Can you work these out from the model? Positions are in its coordinate system, mm. A direction names the side the tool comes from. Coordinates: 2 decimals unless noted, no trailing zeros. Order: outer loops, then holes, each group sorted by start corner. A loop starts at its lowest first (then second) coordinate and runs counter-clockwise, first axis right, second up. Notation, with made-up numbers: (66, -2) -> (108, -2) arc R16 ccw to (108, 5) -> close; hole circle Ø3 at (-32.75, 18). An arc over 180 degrees is marked (long way). Write item = value, one per line.
```python
from build123d import *

# Parameters (mm, degrees)
BOSS_EXTRUDE1_DEPTH = 17
CUT_EXTRUDE1_DEPTH  = 31
SKETCH3_W           = 12.47
SKETCH3_H           = 10.75
CUT_EXTRUDE2_REACH  = 37.239
SKETCH6_W           = 10
SKETCH6_H           = 10.75
SKETCH7_R           = 4
CUT_EXTRUDE3_DEPTH  = 31


with BuildPart() as part:
    # Sketch1 → Boss-Extrude1 (new body)
    with BuildSketch(Plane.XY):
        Polygon((0, 0), (0, 11.1), (5.04, 11.1), (5.04, -5.9), (1.928970145, -13.9), (-4.358645915, -16.03435805), (-26.37555014, -13.036971131), (-26.37555014, 11.1), (-21.33555014, 11.1), (-21.33555014, 0), align=None)
    extrude(amount=BOSS_EXTRUDE1_DEPTH)

    # Sketch2 → Cut-Extrude1 (cut, symmetric)
    with BuildSketch(Plane.ZY):
        Polygon((8.228054067, 11.1), (17, 11.1), (17, 12.88110255), (0, 12.88110255), (0, 11.1), align=None)
        with BuildLine():
            ThreePointArc((0, 0), (2.28131811, 6.908525055), (8.228054067, 11.1))
            Line((8.228054067, 11.1), (0, 11.1))
            Line((0, 11.1), (0, 0))
        make_face()
        Polygon((13.228054067, 10.512247596), (17, 6.76), (17, 11.1), (8.228054067, 11.1), align=None)
    extrude(amount=CUT_EXTRUDE1_DEPTH, both=True, mode=Mode.SUBTRACT)

    # Cut-Sweep1: sweep along a path in Sketch5
    with BuildLine(Plane.XY.offset(7)) as cut_sweep1_path:
        Line((-9.535960256, -15.329517164), (-6.500512954, -6.687083497))
    # Sketch3 → Cut-Sweep1 (sweep, cut)
    with BuildSketch(Plane(origin=(-2.222513014, -16.325171724, 0), x_dir=(-0.990859776111597, 0.13489590091650622, 0), z_dir=(-0.13489590091650622, -0.990859776111597, 0))):
        with Locations((12.41083774, -9.115)):
            Rectangle(SKETCH3_W, SKETCH3_H)
    sweep(path=cut_sweep1_path.line, mode=Mode.SUBTRACT)

    # Cut-Extrude2: up to this plane
    cut_extrude2_end = Plane(origin=(-8.680240671, -16.455383538, 3.74), z_dir=(-0.943497125175066, 0.33138070973788714, 0))
    # Sketch6 → Cut-Extrude2 (cut, up to the surface)
    with BuildSketch(Plane(origin=(0, 0, 0), x_dir=(1, 0, 0), z_dir=(0, 1, 0)), mode=Mode.PRIVATE) as cut_extrude2_sk1:
        with Locations((-8.42, -9.115)):
            Rectangle(SKETCH6_W, SKETCH6_H)
    cut_extrude2_tool1 = split(extrude(cut_extrude2_sk1.sketch, amount=-CUT_EXTRUDE2_REACH, mode=Mode.PRIVATE), bisect_by=cut_extrude2_end, keep=Keep.BOTH, mode=Mode.PRIVATE)
    add(cut_extrude2_tool1.solids().sort_by_distance((-8.42, 0, 9.115))[0], mode=Mode.SUBTRACT)

    # Sketch7 → Cut-Extrude3 (cut, symmetric)
    with BuildSketch(Plane.ZY.offset(10.66777507)):
        with Locations(Location((8.5, 4.041620851, 0), (0, 0, 270))):
            Circle(SKETCH7_R)
    extrude(amount=CUT_EXTRUDE3_DEPTH, both=True, mode=Mode.SUBTRACT)


solid = part.part
```
Item 1: If we mould it in two halves opening along Z, with no side actions, what happens to faces 1 (the flat face through (5.04, -1, 8)), 2 (the cylindrical face through (2.485, 4.909, 4.595)), 3 (the cylindrical face through (2.5, 6.8, 2.2))? For each: pulls with the +Z half, pulls with the -Z half, needs draft (parallel to the pull), parting line crosses it, or undercut.
A:
face_1 = needs draft
face_2 = undercut
face_3 = pulls with the -Z half
Item 2: If I drill on probe 1 along X at (y, z) = (5, 4); probe 2 along X at (y, z) = (-11.5, 10); probe 3 along Y at (x, z) = (-23, 15.25), over which ranges is the centre line in solid material (lowest first)?
A:
probe_1 = -26.38 to -21.34, 0 to 5.04
probe_2 = -26.38 to -19.89, -6.94 to 2.86
probe_3 = -13.5 to 8.5
Item 3: I'm going to push flat-ended pins straight in: P1, Ø9, axis at y = 4.04, z = 8.5, coming from the -X side; P2, Ø1, axis at x = -16.5, z = 15, coming from the -Y side. Where does each tip first touch, or does it pass through?
A:
P1 = -26.38
P2 = -14.45
Item 4: I want a section at B-B, the plane z = 10. Please give me the cut outline in (x, y).
A:
outline = (-26.38, -13.04) -> (-20.7, -13.81) -> (-17.66, -5.17) -> (-13.42, -5.75) -> (-13.42, 0) -> (-21.34, 0) -> (-21.34, 0.33) -> (-26.38, 0.33) -> close; (-26.38, 7.75) -> (-21.34, 7.75) -> (-21.34, 10.89) -> (-26.38, 10.89) -> close; (-8.34, -15.49) -> (-4.36, -16.03) -> (1.93, -13.9) -> (5.04, -5.9) -> (5.04, 0.33) -> (0, 0.33) -> (0, 0) -> (-3.42, 0) -> (-3.42, -1.48) -> close; (0, 7.75) -> (5.04, 7.75) -> (5.04, 10.89) -> (0, 10.89) -> close
Item 5: For faces 4 (the flat face through (-13.42, -3, 9)), 5 (the flat face through (-21.336, 8, 10)), 6 (the flat face through (-12, -8, 3.74)), which set-ups out of +Z, -Z, +X, -X, +Y, -Y let a thin tool reach every point of the face, with its end or its side?
A:
face_4 = +Y, -Y
face_5 = +Z, -Z, +Y
face_6 = none
Item 6: I want a section at D-D, the plane z = 1. Please give me the cut outline in (x, y).
A:
outline = (-26.38, -13.04) -> (-4.36, -16.03) -> (1.93, -13.9) -> (5.04, -5.9) -> (5.04, 4.71) -> (0, 4.71) -> (0, 0) -> (-21.34, 0) -> (-21.34, 4.71) -> (-26.38, 4.71) -> close
Item 7: I want a section at A-A, the plane y = 9. Please give me the cut outline in (x, z).
A:
outline = (-26.38, 4.28) -> (-21.34, 4.28) -> (-21.34, 14.75) -> (-26.38, 14.75) -> close; (0, 4.28) -> (5.04, 4.28) -> (5.04, 14.75) -> (0, 14.75) -> close
Item 8: I want a section at C-C, the plane y = 5.75. Please give me the cut outline in (x, z).
A:
outline = (-26.38, 1.53) -> (-21.34, 1.53) -> (-21.34, 4.88) -> (-26.38, 4.88) -> close; (-26.38, 12.12) -> (-21.34, 12.12) -> (-21.34, 17) -> (-26.38, 17) -> close; (0, 1.53) -> (5.04, 1.53) -> (5.04, 4.88) -> (0, 4.88) -> close; (0, 12.12) -> (5.04, 12.12) -> (5.04, 17) -> (0, 17) -> close
